Read the model definition and answer for the solid it produces. Units are mm, in the model's axes. Face numbers are marked on the shaded views. A direction names the side the tool comes from. Coordinates: 2 decimals unless noted, no trailing zeros. Order: outer loops, then holes, each group sorted by start corner. A loop starts at its lowest first (then second) coordinate and runs counter-clockwise, first axis right, second up. Notation, with made-up numbers: (53.25, 75.25) -> (78.25, 75.25) arc R24 cw to (78.25, 97.25) -> close; hole circle Ø2 at (-31, 74.25). An arc over 180 degrees is marked (long way). Use CSV: the item, a comma, the result in double quotes.
```python
from build123d import *

# Parameters (mm, degrees)
SKETCH1_R           = 8
BOSS_EXTRUDE1_DEPTH = 14
SKETCH2_R           = 9.5
BOSS_EXTRUDE2_DEPTH = 2
SKETCH3_R           = 6.5
BOSS_EXTRUDE3_DEPTH = 4
FILLET1_R           = 2


with BuildPart() as part:
    # Sketch1 → Boss-Extrude1 (new body)
    with BuildSketch(Plane.XY):
        Circle(SKETCH1_R)
    extrude(amount=BOSS_EXTRUDE1_DEPTH)

    # Sketch2 → Boss-Extrude2 (add)
    with BuildSketch(Plane.XY.offset(14)):
        Circle(SKETCH2_R)
    extrude(amount=BOSS_EXTRUDE2_DEPTH)

    # Sketch3 → Boss-Extrude3 (add)
    with BuildSketch(Plane.XY.offset(16)):
        Circle(SKETCH3_R)
    extrude(amount=BOSS_EXTRUDE3_DEPTH)

    # Fillet1
    fillet1_edges = [part.edges().sort_by_distance(p)[0] for p in [
        (-6.5, 0, 20),
    ]]
    fillet(fillet1_edges, radius=FILLET1_R)


solid = part.part
```
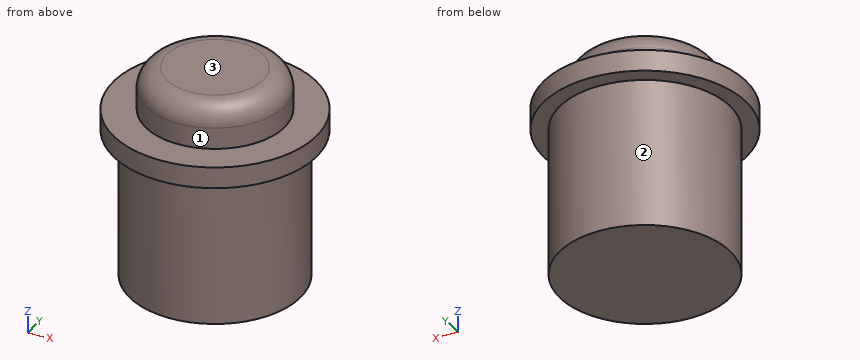
Item 1: Straight lines are drawn through the part: line 1 along Z through (x, y) = (-6, -3.25); line 2 along Z through (x, y) = (3.25, -3.25); line 3 along Y through (x, z) = (-7, 11). For each, find the intervals that lie inside material, in ascending order.
Return value:
line 1,"z = 0 to 16"
line 2,"z = 0 to 20"
line 3,"y = -3.87 to 3.87"
Item 2: Each of these flat-tipped pins is pushed along its axis until it touches: P1, Ø5, axis at y = 5, z = 6, coming from the -X side; P2, Ø2, axis at x = -5.5, z = 8, coming from the +Y side; P3, Ø4, axis at x = -4, z = 13.5, coming from the -Y side. Where does it stop, or does it pass through?
Return value:
P1,"stops at x = -7.6"
P2,"stops at y = 6.61"
P3,"stops at y = -9.27"
Item 3: Find section D-D, the plane x = 7. Give the vertices of the cut face in (y, z).
Return value:
outline,"(-6.42, 14) -> (-3.87, 14) -> (-3.87, 0) -> (3.87, 0) -> (3.87, 14) -> (6.42, 14) -> (6.42, 16) -> (-6.42, 16) -> close"
Item 4: Find section A-A, the plane x = 0. Give the vertices of the cut face in (y, z), then the cut area to 3 significant figures.
Return value:
outline,"(-9.5, 14) -> (-8, 14) -> (-8, 0) -> (8, 0) -> (8, 14) -> (9.5, 14) -> (9.5, 16) -> (6.5, 16) -> (6.5, 18) arc R2 ccw to (4.5, 20) -> (-4.5, 20) arc R2 ccw to (-6.5, 18) -> (-6.5, 16) -> (-9.5, 16) -> close"
area,"312 mm^2"
Item 5: A tool of negligible diameter and unlimited length cuts with its end or side. For the marked faces 1, 2 and 3, from which of +Z, -Z, +X, -X, +Y, -Y can it reach the whole face along a straight path? Write none if from no direction.
Return value:
face 1,"+Z"
face 2,"-Z"
face 3,"+Z, +X, -X, +Y, -Y"
Item 6: Find section C-C, the plane z = 6. Give the vertices of the cut face in (x, y).
Return value:
outline,"circle Ø16 at (0, 0)"
